Autodesk Inventor part; units mm, degrees
ref_plane "YZ Plane" through (0, 0, 0) normal (1, 0, 0) x (0, 1, 0)
ref_plane "XZ Plane" through (0, 0, 0) normal (0, 1, 0) x (-1, 0, 0)
ref_plane "XY Plane" through (0, 0, 0) normal (0, 0, 1) x (1, 0, 0)
sketch "Sketch1" plane through (0, 0, 0) normal (0, 0, 1) x (1, 0, 0)
  line L0 (-19.05, -19.05) -> (19.05, -19.05)
  line L1 (19.05, -19.05) -> (19.05, 19.05)
  line L2 (19.05, 19.05) -> (-19.05, 19.05)
  line L3 (-19.05, 19.05) -> (-19.05, -19.05)
  line L4 (-19.05, -19.05) -> (19.05, 19.05) construction
  line L5 (19.05, -19.05) -> (-19.05, 19.05) construction
  point P0 (0, 0)
  dimension "d0" = 38.1
  dimension "d1" = 38.1
extrude "Extrusion1" add sketch "Sketch1" along normal blind 6.35
sketch "Sketch2" plane through (0, 0, 6.35) normal (0, 0, 1) x (1, 0, 0)
  line L0 (-23.8125, -19.05) -> (23.8125, -19.05)
  line L1 (23.8125, -19.05) -> (23.8125, 19.05)
  line L2 (23.8125, 19.05) -> (-23.8125, 19.05)
  line L3 (-23.8125, 19.05) -> (-23.8125, -19.05)
  line L4 (-23.8125, -19.05) -> (23.8125, 19.05) construction
  line L5 (23.8125, -19.05) -> (-23.8125, 19.05) construction
  point P0 (0, 0)
  point P1 (19.05, 19.05)
  dimension "d4" = 47.625
extrude "Extrusion2" add sketch "Sketch2" along normal blind 2.3813
sketch "Sketch3" plane through (-19.05, 19.05, 0) normal (0, 1, 0) x (1, 0, 0)
  line L0 (0, 0) -> (0, -6.35) construction
  line L1 (0, -6.35) -> (-0.5613, -5.7887) construction
  line L2 (0, -6.35) -> (-4.7625, -6.35) construction
  circle A0 centre (-0.5613, -5.7887) radius 0.7937
  line L3 (19.05, 0) -> (19.05, -8.7313) construction
  line L4 (42.8625, -8.7313) -> (-4.7625, -8.7313)
  circle A1 centre (38.6613, -5.7887) radius 0.7937
  dimension "d8" = 1.5875
  dimension "d7" = 45
extrude "Extrusion3" cut sketch "Sketch3" against normal through all
fillet "Fillet1" radius 3.175 4 edges at (-19.05, 0, 5.2275) (-20.1725, 0, 6.35) (20.1725, 0, 6.35) (19.05, 0, 5.2275)
sketch "Sketch4" plane through (0, 0, 8.7313) normal (0, 0, 1) x (1, 0, 0)
  circle A0 centre (0, 0) radius 4.05
  circle A1 centre (0, 0) radius 8 construction
  circle A2 centre (0, 0) radius 9.5 construction
  line L0 (0, 0) -> (0, 9.5) construction
  line L1 (0, 0) -> (-5.6569, 5.6569) construction
  line L2 (0, 0) -> (-6.7175, -6.7175) construction
  circle A3 centre (-5.6569, 5.6569) radius 1.5
  circle A4 centre (-6.7175, -6.7175) radius 1.5
  circle A5 centre (6.7175, 6.7175) radius 1.5
  circle A6 centre (5.6569, -5.6569) radius 1.5
  dimension "d13" = 16
  dimension "d12" = 8.1
  dimension "d14" = 19
  dimension "d15" = 45
  dimension "d16" = 3
  dimension "d17" = 3
  dimension "d20" = 360
extrude "Extrusion4" cut sketch "Sketch4" against normal through all
chamfer "Chamfer1" distance 1.5875 angle 45 1 edges at (-4.05, 0, 8.7313)
properties part number "Drill Guide"
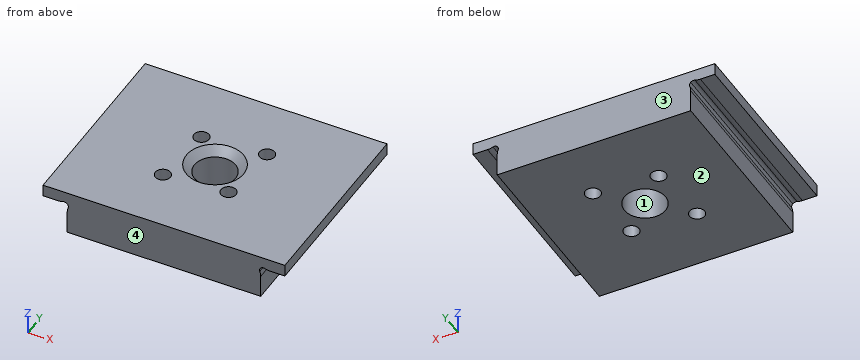
Here's how the part is built. I have some questions about the finished solid (model axes, mm). Face numbers are marked on the shaded views. Round coordinates to 2 decimals unless told otherwise and drop trailing zeros. Loops run counter-clockwise (first coordinate to the right, second up) from the corner with the lowest first, then second, coordinate; pieces in that order, holes last. Notation, with made-up numbers: M -29,76 L -14,76 A15 cw -14,93 Z; hole C 27.5,39.5 d7. An arc over 180 degrees is marked long. Write each question's results on one line, items separated by ' | '. Start each with the question number.
(1) Thinking about a two-plate mould opening in Y: for the marked faces 1, 2, 3 and 4, which applies, pulls with the +Y half, pulls with the -Y half, needs draft (parallel to the pull), parting line crosses it, or undercut?
(2) Will these pins go through, and if not, where does the flat tip stop? P1, Ø1.4, axis at x = -22, y = -3, coming from the -Z side; P2, Ø2, axis at y = 6.5, z = 3, coming from the -X side; P3, Ø4, axis at y = 6, z = 1.5, coming from the +X side; P4, Ø7.5, axis at x = 0, y = 0, coming from the +Z side.
(3) I want a section at C-C (z = 0.5). Please give me the cut outline in (x, y).
(4) If I drill on probe 1 along X at (y, z) = (5.5, 5.75); probe 2 along X at (y, z) = (-5.5, 4.5); probe 3 along Y at (x, z) = (-7, 3.5), over which ranges is the centre line in solid material (lowest first)? Write a range as from..to.
(5) I want a section at A-A (x = 0). Please give me the cut outline in (y, z).
Solved:
1) face 1: undercut | face 2: needs draft | face 3: pulls with the +Y half | face 4: pulls with the -Y half
2) P1: stops at z = 6.35 | P2: stops at x = -19.05 | P3: stops at x = 19.05 | P4: passes through
3) outline: M -19.05,-19.05 L 19.05,-19.05 L 19.05,19.05 L -19.05,19.05 Z; hole C -6.72,-6.72 d3; hole C -5.66,5.66 d3; hole C 0,0 d8.1; hole C 5.66,-5.66 d3; hole C 6.72,6.72 d3
4) probe 1: x = -18.82..-7.15, -4.17..5.84, 7.59..18.82 | probe 2: x = -19.05..-7.59, -5.84..4.17, 7.15..19.05 | probe 3: y = -19.05..-8.19, -5.24..4.99, 6.32..19.05
5) outline: M -19.05,0 L -4.05,0 L -4.05,7.14 L -5.64,8.73 L -19.05,8.73 Z; M 4.05,0 L 19.05,0 L 19.05,8.73 L 5.64,8.73 L 4.05,7.14 Z
